Can you work these out from the model? Positions are in its coordinate system, mm. Face numbers are marked on the shaded views. A direction names the side the tool comes from. Round coordinates to 2 decimals unless told otherwise and drop trailing zeros. Order: outer loops, then holes, each group sorted by start corner. A loop starts at its lowest first (then second) coordinate and runs counter-clockwise, first axis right, second up. Notation, with made-up numbers: (32.25, 6) -> (50.25, 6) arc R27 ccw to (50.25, 23) -> close; hole circle Ø8 at (84, 89.5). An arc over 180 degrees is marked (long way). Use a Markdown table: item, result. Add a question column.
Q1. I'm going to push flat-ended pins straight in: pin 1 Ø10 at (x, z) = (364.5, 16.5) entering from +Y; pin 2 Ø1.5 at (y, z) = (50, 53.5) entering from +X. Where does each tip first touch, or does it pass through?
Q2. If we section it at C-C on y = 109: List the corners of the cut face in (x, z) for me.
Q3. We'd pull the mould along X, two halves only. Please class the marked faces 1, 2 and 3: +X half, -X half, draft (parallel to the pull), parting line (faces both ways), or undercut.
Q4. If we section it at B-B on x = 225.5: List the corners of the cut face in (y, z) for me, plus the area to 3 significant figures.
Q5. If we section it at D-D on y = 85: List the corners of the cut face in (x, z) for me.
Q6. If we section it at A-A on z = 35: List the corners of the cut face in (x, y) for me.
Q7. For the marked faces 4 and 5, which set-ups out of +Z, -Z, +X, -X, +Y, -Y let a thin tool reach every point of the face, with its end or its side?
Q8. I need wall thicknesses on line 1 along Y through (x, z) = (533.5, 30); line 2 along Y through (x, z) = (65, 35); line 3 along Y through (x, z) = (14.5, 30). Which ranges of each line are inside material? Lowest first, please. Write a range as [from, to].
Autodesk Inventor part; units mm, degrees
ref_plane "Plano de trabajo1" through (65, 0, 0) normal (1, 0, 0) x (0, 0, -1)
ref_plane "YZ Plane" through (0, 0, 0) normal (1, 0, 0) x (0, 1, 0)
ref_plane "XZ Plane" through (0, 0, 0) normal (0, 1, 0) x (-1, 0, 0)
sketch "Boceto1" plane through (0, 0, 0) normal (0, 0, 1) x (1, 0, 0)
  line L0 (0, 0) -> (130, 0)
  line L1 (130, 0) -> (130, 95)
  line L2 (130, 95) -> (545, 95)
  line L3 (545, 95) -> (545, 170)
  line L4 (545, 170) -> (0, 170)
  line L5 (0, 170) -> (0, 0)
  circle A0 centre (65, 85) radius 10
  dimension "d1" = 95
  dimension "d3" = 75
  dimension "d19" = 20
extrude "Extrusión1" add sketch "Boceto1" along normal blind 60 contours L5 L4 L3 L2 L1 L0 | A0
ref_plane "Plano de trabajo1" through (65, 0, 0) normal (1, 0, 0) x (0, 0, -1)
sketch "Boceto2" plane through (65, 0, 0) normal (1, 0, 0) x (0, 0, -1)
  line L0 (-20, 75) -> (-40, 75)
  line L1 (-40, 75) -> (-40, 20)
  line L2 (0, 0) -> (-60, 0)
  line L3 (-40, 20) -> (-20, 20)
  line L4 (-20, 75) -> (-20, 20)
  dimension "d8" = 20
  dimension "d9" = 55
  dimension "d10" = 20
extrude "Extrusión2" cut sketch "Boceto2" along normal blind 400 and the other way blind 200
sketch "Boceto3" plane through (130, 0, 0) normal (1, 0, 0) x (0, 0, -1)
  line L0 (-20, 75) -> (-40, 75)
  line L1 (-40, 75) -> (-40, 150)
  line L2 (0, 170) -> (-60, 170)
  line L3 (-40, 150) -> (-20, 150)
  line L4 (-20, 150) -> (-20, 75)
  point P0 (0, 0)
  dimension "d15" = 75
  dimension "d16" = 20
extrude "Extrusión3" cut sketch "Boceto3" along normal mid plane 7000
sketch "Boceto4" plane through (65, 0, 0) normal (1, 0, 0) x (0, 0, -1)
  point P0 (0, 0)
sketch "Boceto5" plane through (0, 0, 60) normal (0, 0, 1) x (1, 0, 0)
  line L0 (130, 95) -> (545, 95)
  line L1 (545, 170) -> (0, 170)
  line L2 (0, 0) -> (130, 0)
  point P0 (65, 85)
hole "Agujero1" at (65, 85, 60) direction (0, 0, -1) diameter 0.2159 end through all
sketch "Boceto6" plane through (0, 0, 0) normal (-1, 0, 0) x (0, 0, 1)
  line L0 (0, 170) -> (0, 0)
  line L1 (40, 95) -> (60, 95)
  line L2 (0, 95) -> (60, 95)
  line L3 (0, 95) -> (0, 170)
  line L4 (0, 170) -> (60, 170)
  line L5 (60, 170) -> (60, 95)
extrude "Extrusión4" add sketch "Boceto6" against normal blind 20
ref_plane "Plano de trabajo8" through (272.5, 0, 0) normal (-1, 0, 0) x (0, 0, 1)
sketch "Boceto7" plane through (272.5, 0, 0) normal (-1, 0, 0) x (0, 0, 1)
  line L0 (40, 95) -> (60, 95)
  line L1 (0, 75) -> (0, 95)
  line L2 (60, 95) -> (0, 95)
  line L3 (0, 95) -> (0, 170)
  line L4 (0, 170) -> (60, 170)
  line L5 (60, 0) -> (60, 95)
  line L6 (60, 170) -> (60, 95)
  point P0 (0, 0)
extrude "Extrusión5" add sketch "Boceto7" against normal blind 273
sketch "Boceto8" plane through (130, 95, 0) normal (0, -1, 0) x (1, 0, 0)
  line L0 (-130, 60) -> (415.5, 60)
  line L1 (415.5, 0) -> (415.5, 60)
  line L2 (395.5, 40) -> (395.5, 20)
  line L3 (0, 0) -> (415.5, 0)
  line L4 (395.5, 40) -> (142.5, 40)
  line L5 (142.5, 20) -> (0, 20)
  line L6 (142.5, 40) -> (142.5, 20)
  line L7 (142.5, 20) -> (395.5, 20)
  point P0 (-130, 0)
  point P1 (415, 60)
  point P2 (415, 0)
  point P3 (415, 20)
  dimension "d35" = 20
extrude "Extrusión6" cut sketch "Boceto8" against normal blind 75
sketch "Boceto9" plane through (130, 95, 0) normal (0, -1, 0) x (1, 0, 0)
  line L0 (142.5, 20) -> (142.5, 40)
  line L1 (142.5, 20) -> (142.5, 40)
  line L2 (142.5, 40) -> (1, 40)
  line L3 (1, 40) -> (1, 20)
  line L4 (142.5, 20) -> (-110, 20)
  line L5 (1, 20) -> (142.5, 20)
  point P0 (-130, 0)
extrude "Extrusión7" cut sketch "Boceto9" against normal blind 75
sketch "Boceto10" plane through (0, 0, 60) normal (0, 0, 1) x (1, 0, 0)
  point P0 (0, 0)
ref_plane "Plano de trabajo9" through (535.5, 0, 0) normal (1, 0, 0) x (0, 0, -1)
sketch "Boceto11" plane through (545.5, 0, 0) normal (1, 0, 0) x (0, 0, -1)
  line L0 (0, 95) -> (-20, 95)
  line L1 (0, 170) -> (-60, 170)
  line L2 (0, 95) -> (-60, 170)
  line L3 (-60, 84.892) -> (-60, 85.108)
  line L4 (0, 170) -> (-60, 85.108)
  circle A0 centre (-30, 127.554) radius 10
  point P0 (0, 0)
  dimension "d40" = 20
hole "Agujero2" at (545.5, 127.554, 30) direction (-1, 0, 0) diameter 20 end through all
sketch "Boceto12" plane through (0, 0, 60) normal (0, 0, 1) x (1, 0, 0)
  line L0 (0, 170) -> (0, 0)
  line L1 (130, 0) -> (130, 95)
  line L2 (0, 170) -> (130, 0)
  line L3 (130, 95) -> (130, 170)
  line L4 (130, 170) -> (0, 0)
  circle A0 centre (65, 85) radius 10
  dimension "d48" = 20
hole "Agujero3" at (65, 85, 60) direction (0, 0, -1) diameter 20 end through all
extrude "Extrusión8" [suppressed]
hole "Agujero4" at (65, 85, 60) direction (0, 0, -1) diameter 17.8943 end through all
sketch "Boceto13" plane through (0, 170, 60) normal (0, 1, 0) x (1, 0, 0)
  line L0 (131, 40) -> (131, 50)
  line L1 (525.5, 20) -> (525.5, 40)
  line L2 (525.5, 40) -> (525.5, 50)
  line L3 (525.5, 50) -> (131, 50)
  line L4 (131, 40) -> (525.5, 40)
  line L5 (131, 40) -> (525.5, 40)
  line L6 (525.5, 20) -> (131, 20)
  line L7 (131, 20) -> (131, 10)
  line L8 (525.5, 20) -> (525.5, 10)
  line L9 (525.5, 10) -> (131, 10)
  point P0 (0, 60)
  dimension "d65" = 10
  dimension "d66" = 10
  dimension "d67" = 10
  dimension "d68" = 10
extrude "Extrusión9" cut sketch "Boceto13" against normal through all
sketch "Boceto14" plane through (130, 20, 40) normal (0, 0, -1) x (-1, 0, 0)
  circle A0 centre (65, 65) radius 10
  circle A1 centre (65, 65) radius 10
  point P0 (130, -20)
extrude "Extrusión10" add sketch "Boceto14" along normal blind 40
sketch "Boceto15" plane through (0, 0, 60) normal (0, 0, 1) x (1, 0, 0)
  circle A0 centre (65, 85) radius 10
  circle A1 centre (65, 85) radius 18.123
  point P0 (0, 0)
  dimension "d80" = 36.246
hole "Agujero5" at (65, 85, 60) direction (0, 0, -1) diameter 36.2458 end through all
extrude "Extrusión11" add sketch "Boceto15" along normal mid plane 150 contours A0 | A1
sketch "Boceto16" plane through (0, 0, 0) normal (0, -1, 0) x (1, 0, 0)
  line L0 (0, 60) -> (0, 142)
  line L1 (130, 40) -> (130, 60)
  line L2 (130, 60) -> (130, 150)
  line L3 (130, 150) -> (0, 142)
  line L4 (0, 60) -> (130, 60)
  line L5 (131, 50) -> (525.5, 50)
  point P0 (0, 0)
extrude "Extrusión12" cut sketch "Boceto16" against normal blind 150
sketch "Boceto17" plane through (0, 170, 60) normal (0, 1, 0) x (1, 0, 0)
  line L0 (0, 60) -> (130, 60)
  line L1 (0, 60) -> (0, 117)
  line L2 (130, 60) -> (130, 106)
  line L3 (0, 60) -> (130, 60)
  line L4 (0, 117) -> (130, 106)
extrude "Extrusión13" cut sketch "Boceto17" against normal blind 150
sketch "Boceto18" plane through (0, 0, 60) normal (0, 0, 1) x (1, 0, 0)
  circle A0 centre (65, 85) radius 10
  point P0 (0, 0)
  dimension "d87" = 20
hole "Agujero6" at (65, 85, 60) direction (0, 0, -1) diameter 0.2159 end through all
hole "Agujero7" at (65, 85, 60) direction (0, 0, -1) diameter 20 end through all
thread "Rosca1"
properties part number "PiezaMovil"
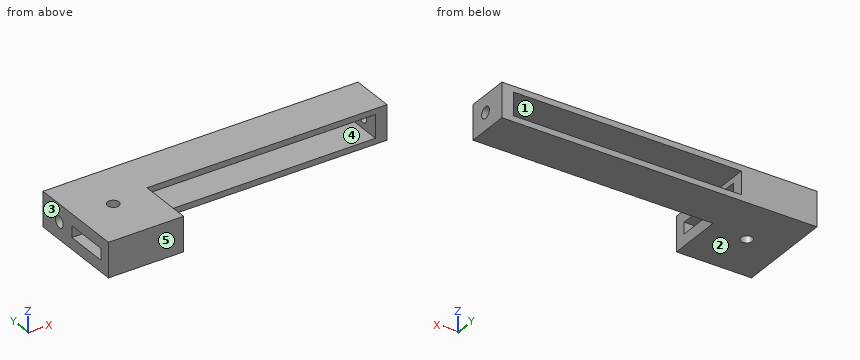
Answer below:
| question | item | result |
|---|---|---|
| 1 | pin 1 | through |
| 1 | pin 2 | x = 130 |
| 2 | outline | (0, 0) -> (545.5, 0) -> (545.5, 60) -> (0, 60) -> close; hole (20, 20) -> (131, 20) -> (131, 10) -> (525.5, 10) -> (525.5, 50) -> (131, 50) -> (131, 40) -> (20, 40) -> close |
| 3 | face 1 | undercut |
| 3 | face 2 | draft |
| 3 | face 3 | -X half |
| 4 | outline | (95, 0) -> (170, 0) -> (170, 10) -> (95, 10) -> close; (95, 50) -> (170, 50) -> (170, 60) -> (95, 60) -> close |
| 4 | area | 1,500 mm² |
| 5 | outline | (0, 0) -> (55, 0) -> (55, 60) -> (0, 60) -> (0, 40) -> (46.88, 40) -> (46.88, 20) -> (0, 20) -> close; (75, 0) -> (130, 0) -> (130, 20) -> (83.12, 20) -> (83.12, 40) -> (130, 40) -> (130, 60) -> (75, 60) -> close |
| 6 | outline | (0, 0) -> (130, 0) -> (130, 20) -> (0, 20) -> close; (0, 95) -> (20, 95) -> (20, 118.89) -> (0, 118.89) -> close; (0, 136.21) -> (20, 136.21) -> (20, 150) -> (131, 150) -> (131, 170) -> (0, 170) -> close; circle Ø36.25 at (65, 85); (525.5, 95) -> (545.5, 95) -> (545.5, 118.89) -> (525.5, 118.89) -> close; (525.5, 136.21) -> (545.5, 136.21) -> (545.5, 170) -> (525.5, 170) -> close; hole circle Ø20 at (65, 85) |
| 7 | face 4 | +Y, -Y |
| 7 | face 5 | +Z, -Z, +X, -X, -Y |
| 8 | line 1 | [95, 117.55], [137.55, 170] |
| 8 | line 2 | [0, 20], [66.88, 75], [95, 103.12], [150, 170] |
| 8 | line 3 | [0, 20], [95, 117.55], [137.55, 170] |
